Read the model definition and answer for the solid it produces. Units are mm, in the model's axes. A direction names the side the tool comes from. Coordinates: 2 decimals unless noted, no trailing zeros. Write each loop counter-clockwise with the first axis right and the second up, starting at its lowest first coordinate (ties: lowest second). Pieces come first, ordered by that corner, then holes.
1) Find the intervals of material crossed by line 1 (X direction, y = 2.05, z = -7.5); line 2 (X direction, y = 2.35, z = -75); line 3 (Z direction, x = -6, y = 2.75), in increasing order.
2) Which of the six approach directions +Z, -Z, +X, -X, +Y, -Y give full straight-line access (tool end or side, diameter ignored) to faces 5 (the face through (18.744, 2, -6)), 6 (the face through (7, 2, 13.416)), 7 (the face through (16, 2, -85.234))?
3) Determine the mould class of faces 1 (the face through (80, 2, -91.584)), 2 (the face through (64.466, 1.565, -45.504)), 3 (the face through (28.253, 1.565, -56.515)), 4 (the face through (-5, 3.175, -16)) for opening direction Z: +Z half, -Z half, draft (parallel to the pull), parting line (faces both ways), or undercut.
4) Each of these flat-tipped pins is pushed along its axis until it touches: pin 1 Ø0.6 at (x, y) = (18, 1) entering from -Z; pin 2 Ø1.7 at (x, z) = (-27.62, -32.39) entering from -Y; pin 3 Ø1 at (x, y) = (-34.5, 2) entering from +Z. Where does it stop, or does it pass through?
5) The part is cut by section A-A (x = -73). Determine the outline of the cut face in (y, z) (3 decimals), then the cut area to 3 significant figures.
6) The part is cut by section B-B (y = 1.2). Give the number of separate pieces and of enclosed holes in the cut face, then the cut area to 3 significant figures.
from build123d import *

# Parameters (mm, degrees)
SKETCH1_R      = 1.9
SKETCH1_R_2    = 1.58353158
SKETCH1_R_3    = 1.50705101
SKETCH1_R_4    = 1.0795
SKETCH1_W      = 32.345315457
SKETCH1_H      = 30
EXTRUDE1_DEPTH = 3.175


with BuildPart() as part:
    # Sketch1 → Extrude1 (new body)
    with BuildSketch(Plane(origin=(0, 0, 0), x_dir=(1, 0, 0), z_dir=(0, 1, 0))):
        Polygon((-67.158636898, 70.484310302), (-67.158636898, 74.492800404), (-68.408636898, 74.492800404), (-68.408636898, 76.742800404), (-67.158636898, 76.742800404), (-67.158636898, 85.234310302), (-82.88813161, 85.234310302), (-82.88813161, 91.584310302), (-92.88813161, 91.584310302), (-92.88813161, -13.415689698), (-82.88813161, -13.415689698), (-82.88813161, -7.065689698), (-67.158636898, -7.065689698), (-67.158636898, 1.425820201), (-68.408636898, 1.425820201), (-68.408636898, 3.675820201), (-67.158636898, 3.675820201), (-67.158636898, 7.684310302), (-64.258636898, 7.684310302), (-64.258636898, 3.675820201), (-63.008636898, 3.675820201), (-63.008636898, 1.425820201), (-64.258636898, 1.425820201), (-64.258636898, -7.065689698), (2.20186839, -7.065689698), (2.20186839, -13.415689698), (12.20186839, -13.415689698), (12.20186839, -7.065689698), (18.744143558, -7.065689698), (18.744143558, 1.771032224), (17.494143558, 1.771032224), (17.494143558, 4.021032224), (18.744143558, 4.021032224), (18.744143558, 7.684310302), (21.644143558, 7.684310302), (21.644143558, 4.021032224), (22.894143558, 4.021032224), (22.894143558, 1.771032224), (21.644143558, 1.771032224), (21.644143558, -7.065689698), (74.914143558, -7.065689698), (74.914143558, -13.415689698), (84.914143558, -13.415689698), (84.914143558, 91.584310302), (74.914143558, 91.584310302), (74.914143558, 85.234310302), (21.644143558, 85.234310302), (21.644143558, 76.397588381), (22.894143558, 76.397588381), (22.894143558, 74.147588381), (21.644143558, 74.147588381), (21.644143558, 70.484310302), (18.744143558, 70.484310302), (18.744143558, 74.147588381), (17.494143558, 74.147588381), (17.494143558, 76.397588381), (18.744143558, 76.397588381), (18.744143558, 85.234310302), (12.20186839, 85.234310302), (12.20186839, 91.584310302), (2.20186839, 91.584310302), (2.20186839, 85.234310302), (-64.258636898, 85.234310302), (-64.258636898, 76.742800404), (-63.008636898, 76.742800404), (-63.008636898, 74.492800404), (-64.258636898, 74.492800404), (-64.258636898, 70.484310302), align=None)
        with Locations(Location((79.354143558, 39.084310302, 0), (0, 0, 270))):
            Circle(SKETCH1_R, mode=Mode.SUBTRACT)
        with Locations(Location((65.194143558, 30.909030491, 0), (0, 0, 270))):
            Circle(SKETCH1_R, mode=Mode.SUBTRACT)
        with Locations(Location((65.194143558, 47.259590114, 0), (0, 0, 270))):
            Circle(SKETCH1_R, mode=Mode.SUBTRACT)
        with Locations(Location((27.777428137, 58.025608002, 0), (0, 0, 270))):
            Circle(SKETCH1_R_2, mode=Mode.SUBTRACT)
        with Locations(Location((78.577377337, 14.845608002, 0), (0, 0, 270))):
            Circle(SKETCH1_R_3, mode=Mode.SUBTRACT)
        with Locations(Location((27.777428137, 30.085608002, 0), (0, 0, 270))):
            Circle(SKETCH1_R_4, mode=Mode.SUBTRACT)
        with Locations(Location((-78.42302428, 17.147481819, 0), (0, 0, 270))):
            Circle(SKETCH1_R_3, mode=Mode.SUBTRACT)
        with Locations(Location((-27.62307508, 32.387481819, 0), (0, 0, 270))):
            Circle(SKETCH1_R_4, mode=Mode.SUBTRACT)
        with Locations(Location((-27.62307508, 60.327481819, 0), (0, 0, 270))):
            Circle(SKETCH1_R_2, mode=Mode.SUBTRACT)
        with Locations((-5.646064502, 40.784310302)):
            Rectangle(SKETCH1_W, SKETCH1_H, mode=Mode.SUBTRACT)
    extrude(amount=EXTRUDE1_DEPTH)


solid = part.part
Reported:
1. line 1: x = -92.89 to -67.16, -64.26 to 18.74, 21.64 to 84.91
1. line 2: x = -92.89 to -68.41, -63.01 to 17.49, 22.89 to 84.91
1. line 3: z = -85.23 to -55.78, -25.78 to 7.07
2. face 5: +Z, +Y, -Y
2. face 6: +Z, +X, -X, +Y, -Y
2. face 7: -Z, +Y, -Y
3. face 1: -Z half
3. face 2: undercut
3. face 3: undercut
3. face 4: draft
4. pin 1: stops at z = -85.23
4. pin 2: passes through
4. pin 3: stops at z = 7.07
5. outline: (0, -85.234) - (3.175, -85.234) - (3.175, 7.066) - (0, 7.066) - close
5. area: 293 mm2
6. separate pieces: 1
6. enclosed holes: 10
6. area: 15,600 mm2
